```python
from build123d import *

# Parameters (mm, degrees)
SKETCH1_W                                       = 40.64
SKETCH1_H                                       = 66.04
SKETCH1_R                                       = 2.5527
SKETCH1_R_2                                     = 2.5908
SKETCH1_R_3                                     = 2.286
SKETCH1_R_4                                     = 2.2479
SKETCH1_R_5                                     = 1.89865
SKETCH1_R_6                                     = 1.9304
SKETCH1_R_7                                     = 1.75
SKETCH1_R_8                                     = 1.7
SKETCH1_R_9                                     = 1.1
SKETCH1_R_10                                    = 1.25
SKETCH1_R_11                                    = 2.5273
SKETCH1_R_12                                    = 2.1971
SKETCH1_R_13                                    = 1.8669
SKETCH1_R_14                                    = 1.15
SKETCH1_R_15                                    = 1.65
BOSS_EXTRUDE1_DEPTH                             = 7.9375
LPATTERN1_COUNT                                 = 2
LPATTERN1_PITCH                                 = 38.1
CBORE_FOR_10_SOCKET_HEAD_CAP_SCREW1_D           = 4.9784
CBORE_FOR_10_SOCKET_HEAD_CAP_SCREW1_CBORE_D     = 9.525
CBORE_FOR_10_SOCKET_HEAD_CAP_SCREW1_CBORE_DEPTH = 4.826
CBORE_FOR_8_SOCKET_HEAD_CAP_SCREW1_D            = 4.3053
CBORE_FOR_8_SOCKET_HEAD_CAP_SCREW1_CBORE_D      = 7.9375
CBORE_FOR_8_SOCKET_HEAD_CAP_SCREW1_CBORE_DEPTH  = 4.1656
CBORE_FOR_6_SOCKET_HEAD_CAP_SCREW1_D            = 3.6576
CBORE_FOR_6_SOCKET_HEAD_CAP_SCREW1_CBORE_D      = 7.14502
CBORE_FOR_6_SOCKET_HEAD_CAP_SCREW1_CBORE_DEPTH  = 3.5052
CBORE_FOR_M3_SHCS1_D                            = 3.2
CBORE_FOR_M3_SHCS1_CBORE_D                      = 6.5
CBORE_FOR_M3_SHCS1_CBORE_DEPTH                  = 3
CBORE_FOR_M2_SHCS1_D                            = 2.2
CBORE_FOR_M2_SHCS1_CBORE_D                      = 4.4
CBORE_FOR_M2_SHCS1_CBORE_DEPTH                  = 2
FILLET1_R                                       = 7.62


with BuildPart() as part:
    # Sketch1 → Boss-Extrude1 (new body)
    with BuildSketch(Plane(origin=(0, 0, 0), x_dir=(1, 0, 0), z_dir=(0, 1, 0))):
        with Locations((20.32, 33.02)):
            Rectangle(SKETCH1_W, SKETCH1_H)
        with Locations(Location((20.32, 58.42, 0), (0, 0, 270))):
            Circle(SKETCH1_R, mode=Mode.SUBTRACT)
        with Locations(Location((33.02, 58.42, 0), (0, 0, 270))):
            Circle(SKETCH1_R_2, mode=Mode.SUBTRACT)
        with Locations(Location((33.02, 45.72, 0), (0, 0, 270))):
            Circle(SKETCH1_R_3, mode=Mode.SUBTRACT)
        with Locations(Location((20.32, 45.72, 0), (0, 0, 270))):
            Circle(SKETCH1_R_4, mode=Mode.SUBTRACT)
        with Locations(Location((20.32, 33.02, 0), (0, 0, 270))):
            Circle(SKETCH1_R_5, mode=Mode.SUBTRACT)
        with Locations(Location((33.02, 33.02, 0), (0, 0, 270))):
            Circle(SKETCH1_R_6, mode=Mode.SUBTRACT)
        with Locations(Location((33.02, 20.32, 0), (0, 0, 270))):
            Circle(SKETCH1_R_7, mode=Mode.SUBTRACT)
        with Locations(Location((20.32, 20.32, 0), (0, 0, 270))):
            Circle(SKETCH1_R_8, mode=Mode.SUBTRACT)
        with Locations(Location((20.32, 7.62, 0), (0, 0, 270))):
            Circle(SKETCH1_R_9, mode=Mode.SUBTRACT)
        with Locations(Location((33.02, 7.62, 0), (0, 0, 270))):
            Circle(SKETCH1_R_10, mode=Mode.SUBTRACT)
        with Locations(Location((7.62, 58.42, 0), (0, 0, 270))):
            Circle(SKETCH1_R_11, mode=Mode.SUBTRACT)
        with Locations(Location((7.62, 45.72, 0), (0, 0, 270))):
            Circle(SKETCH1_R_12, mode=Mode.SUBTRACT)
        with Locations(Location((7.62, 33.02, 0), (0, 0, 270))):
            Circle(SKETCH1_R_13, mode=Mode.SUBTRACT)
        with Locations(Location((7.62, 7.62, 0), (0, 0, 270))):
            Circle(SKETCH1_R_14, mode=Mode.SUBTRACT)
        with Locations(Location((7.62, 20.32, 0), (0, 0, 270))):
            Circle(SKETCH1_R_15, mode=Mode.SUBTRACT)
    extrude(amount=-BOSS_EXTRUDE1_DEPTH)


with BuildPart() as lpattern1_1:
    # LPattern1: pattern copy
    add(part.part.moved(Location(Vector(1, 0, 0) * (1 * LPATTERN1_PITCH))))

    # Combine1: union part
    add(part.part)

    # CBORE for _10 Socket Head Cap Screw1 (through all)
    with Locations(Plane(origin=(0, 0, 0), x_dir=(1, 0, 0), z_dir=(0, 1, 0))):
        with Locations((7.62, 58.42), (20.32, 58.42), (33.02, 58.42)):
            CounterBoreHole(CBORE_FOR_10_SOCKET_HEAD_CAP_SCREW1_D / 2, CBORE_FOR_10_SOCKET_HEAD_CAP_SCREW1_CBORE_D / 2, CBORE_FOR_10_SOCKET_HEAD_CAP_SCREW1_CBORE_DEPTH)

    # CBORE for _8 Socket Head Cap Screw1 (through all)
    with Locations(Plane(origin=(0, 0, 0), x_dir=(1, 0, 0), z_dir=(0, 1, 0))):
        with Locations((7.62, 45.72), (20.32, 45.72), (33.02, 45.72)):
            CounterBoreHole(CBORE_FOR_8_SOCKET_HEAD_CAP_SCREW1_D / 2, CBORE_FOR_8_SOCKET_HEAD_CAP_SCREW1_CBORE_D / 2, CBORE_FOR_8_SOCKET_HEAD_CAP_SCREW1_CBORE_DEPTH)

    # CBORE for _6 Socket Head Cap Screw1 (through all)
    with Locations(Plane(origin=(0, 0, 0), x_dir=(1, 0, 0), z_dir=(0, 1, 0))):
        with Locations((7.62, 33.02), (20.32, 33.02), (33.02, 33.02)):
            CounterBoreHole(CBORE_FOR_6_SOCKET_HEAD_CAP_SCREW1_D / 2, CBORE_FOR_6_SOCKET_HEAD_CAP_SCREW1_CBORE_D / 2, CBORE_FOR_6_SOCKET_HEAD_CAP_SCREW1_CBORE_DEPTH)

    # CBORE for M3 SHCS1 (through all)
    with Locations(Plane(origin=(0, 0, 0), x_dir=(1, 0, 0), z_dir=(0, 1, 0))):
        with Locations((7.62, 20.32), (20.32, 20.32), (33.02, 20.32)):
            CounterBoreHole(CBORE_FOR_M3_SHCS1_D / 2, CBORE_FOR_M3_SHCS1_CBORE_D / 2, CBORE_FOR_M3_SHCS1_CBORE_DEPTH)

    # CBORE for M2 SHCS1 (through all)
    with Locations(Plane(origin=(0, 0, 0), x_dir=(1, 0, 0), z_dir=(0, 1, 0))):
        with Locations((7.62, 7.62), (20.32, 7.62), (33.02, 7.62)):
            CounterBoreHole(CBORE_FOR_M2_SHCS1_D / 2, CBORE_FOR_M2_SHCS1_CBORE_D / 2, CBORE_FOR_M2_SHCS1_CBORE_DEPTH)

    # Fillet1
    fillet1_edges = [lpattern1_1.edges().sort_by_distance(p)[0] for p in [
        (0, -3.96875, -66.04),
    ]]
    fillet(fillet1_edges, radius=FILLET1_R)


solid = lpattern1_1.part
```
Input: part model. Units: mm. Frame: model coordinates. A direction names the side the tool comes from. Coordinates: 2 decimals unless noted, no trailing zeros. Loops run counter-clockwise (first coordinate to the right, second up) from the corner with the lowest first, then second, coordinate; pieces in that order, holes last. Notation, with made-up numbers: M 29,-22.5 L 62,-22.5 A22 cw 62,15.5 Z; hole C 40.5,37.25 d11. An arc over 180 degrees is marked long. One line per item, written item: value.
(1) Line query: line 1 along Z through (x, y) = (58.5, -4.75); line 2 along Z through (x, y) = (34.5, -6.25); line 3 along Z through (x, y) = (8, -0.5). Output: solid intervals per line, ascending. Write a range as from..to.
Filled in:
line 1: -66.04..-60.97, -55.87..-47.97, -43.47..-34.92, -31.12..-22.02, -18.62..-8.72, -6.52..0
line 2: -66.04..-60.55, -56.29..-47.46, -43.98..-34.26, -31.78..-21.25, -19.39..0
line 3: -66.04..-63.17, -53.67..-49.67, -41.77..-36.57, -29.47..-23.55, -17.09..-9.79, -5.45..0
(2) Section B-B (z = -45.72). Give the number of separate pieces and of enclosed holes in the cut face, and give its area (3 significant figures).
Filled in:
separate pieces: 7
enclosed holes: 0
area: 368 mm^2
(3) Reachability of faces 3 (the cylindrical face through (60.02, -3.91, -32)), 4 (the cylindrical face through (17.687, -1.728, -35.434)) from +Z, -Z, +X, -X, +Y, -Y: full face, straight path, thin tool, end or side. Return the list, or none.
Filled in:
face 3: +Y, -Y
face 4: +Y
(4) Section C-C (x = 45.72). Output: boundary loops of the cut face in (y, z), and give its area (3 significant figures).
Filled in:
outline: M -7.94,-66.04 L 0,-66.04 L 0,-60.95 L -7.94,-60.95 Z; M -7.94,-55.89 L 0,-55.89 L 0,-47.92 L -7.94,-47.92 Z; M -7.94,-43.52 L 0,-43.52 L 0,-34.89 L -7.94,-34.89 Z; M -7.94,-31.15 L 0,-31.15 L 0,-21.97 L -7.94,-21.97 Z; M -7.94,-18.67 L 0,-18.67 L 0,-8.77 L -7.94,-8.77 Z; M -7.94,-6.47 L 0,-6.47 L 0,0 L -7.94,0 Z
area: 375 mm^2
(5) Pull-direction query (Z, two-part tool) for faces 1 (the cylindrical face through (7.197, -1.479, -23.542)), 2 (the flat face through (39, -7.938, -33)); classes: +Z half, -Z half, draft (parallel to the pull), parting line (faces both ways), or undercut.
Filled in:
face 1: undercut
face 2: draft
(6) Section D-D (z = -54.5). Output: boundary loops of the cut face in (x, y), and give its area (3 significant figures).
Filled in:
outline: M 0,-7.94 L 78.74,-7.94 L 78.74,0 L 35.72,0 L 35.72,-4.83 L 30.32,-4.83 L 30.32,0 L 23.02,0 L 23.02,-4.83 L 17.62,-4.83 L 17.62,0 L 10.32,0 L 10.32,-4.83 L 4.92,-4.83 L 4.92,0 L 0,0 Z
area: 547 mm^2
(7) Pin query (flat end, axial travel): pin 1 (3 mm diameter, centred on x = 33.02, z = -7.62, fed in from +Y); pin 2 (4 mm diameter, centred on x = 6.5, z = -44.5, fed in from +Y); pin 3 (4.5 mm diameter, centred on x = 20.32, z = -20.32, fed in from +Y). Return the tip coordinate at first contact, or that it passes through.
Filled in:
pin 1: y = -2
pin 2: y = -4.17
pin 3: y = -3
(8) Section A-A (x = 71.12). Output: boundary loops of the cut face in (y, z), and give its area (3 significant figures).
Filled in:
outline: M -7.94,-66.04 L 0,-66.04 L 0,-61.01 L -7.94,-61.01 Z; M -7.94,-55.83 L 0,-55.83 L 0,-48.01 L -7.94,-48.01 Z; M -7.94,-43.43 L 0,-43.43 L 0,-34.95 L -7.94,-34.95 Z; M -7.94,-31.09 L 0,-31.09 L 0,-22.07 L -7.94,-22.07 Z; M -7.94,-18.57 L 0,-18.57 L 0,-8.87 L -7.94,-8.87 Z; M -7.94,-6.37 L 0,-6.37 L 0,0 L -7.94,0 Z
area: 369 mm^2
